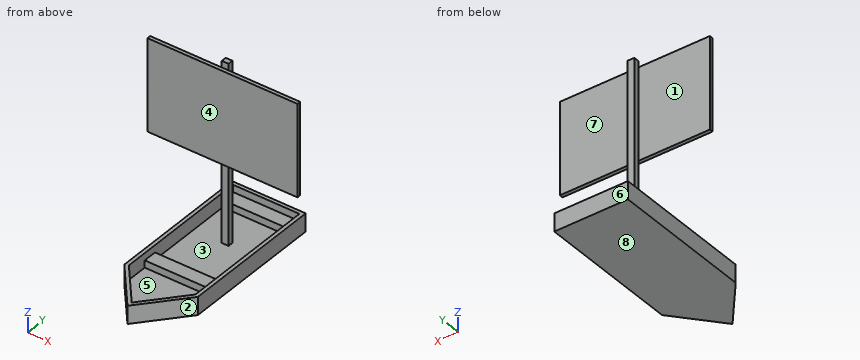
```python
from build123d import *

# Parameters (mm, degrees)
F0_W      = 25.5351066589
F0_H      = 25.5351066589
F0_H_2    = 76.037876308
F0_W_2    = 26.6699995846
F1_DEPTH  = 12.7
F2_T      = -2.54
F3_W      = 47.1251062435
F3_H      = 9.6601096606
F3_H_2    = 9.6465954557
F4_DEPTH  = 5.08
F5_W      = 4.8232972622
F5_H      = 3.6884061992
F6_DEPTH  = 127
F7_W      = 4.8232972622
F7_H      = 2.9607340693
F8_DEPTH  = 2.54
F9_W      = 2.54
F9_H      = 2.9607340693
F10_DEPTH = 50.8
F11_W     = 2.54
F11_H     = 2.9607340693
F12_DEPTH = 50.8
F13_W     = 106.4232972622
F13_H     = 2.54
F14_DEPTH = 62.23


with BuildPart() as f1:
    # F0 (on Top) → F1 (new body)
    with BuildSketch(Plane.XY):
        with Locations((-12.7675533295, -12.7675533295)):
            Rectangle(F0_W, F0_H)
        with Locations((-12.7675533295, 38.018938154)):
            Rectangle(F0_W, F0_H_2)
        with Locations((13.3349997923, 38.018938154)):
            Rectangle(F0_W_2, F0_H_2)
        with Locations((13.3349997923, -12.7675533295)):
            Rectangle(F0_W_2, F0_H)
        Polygon((26.6699995846, -25.5351066589), (0, -25.5351066589), (-25.5351066589, -25.5351066589), (0, -56.4609579742), align=None)
    extrude(amount=F1_DEPTH)

    # F2
    f2_openings = [f1.faces().sort_by_distance(p)[0] for p in [
        (0.542456, 17.179425, 12.7),
    ]]
    offset(amount=F2_T, openings=f2_openings)

    # F3 (on face) → F4 (join)
    with BuildSketch(Plane.XY.offset(2.54)):
        with Locations((0.5674464628, 68.6678214777)):
            Rectangle(F3_W, F3_H)
        with Locations((0.5674464628, -4.8232977279)):
            Rectangle(F3_W, F3_H_2)
    extrude(amount=F4_DEPTH)

    # F5 (on face) → F6 (join)
    with BuildSketch(Plane.XY.offset(2.54)):
        with Locations((-0.1418609172, 37.5933516771)):
            Rectangle(F5_W, F5_H)
    extrude(amount=F6_DEPTH)

    # F7 (on face) → F8 (join)
    with BuildSketch(Plane.XZ.offset(-35.7491485775)):
        with Locations((-0.1418609172, 61.2260736525)):
            Rectangle(F7_W, F7_H)
    extrude(amount=F8_DEPTH)

    # F9 (on face) → F10 (join)
    with BuildSketch(Plane.YZ.offset(2.2697877139)):
        with Locations((34.4791485775, 61.2260736525)):
            Rectangle(F9_W, F9_H)
    extrude(amount=F10_DEPTH)

    # F11 (on face) → F12 (join)
    with BuildSketch(Plane(origin=(-2.5535095483, 0, 0), x_dir=(0, -1, 0), z_dir=(-1, 0, 0))):
        with Locations((-34.4791485775, 61.2260736525)):
            Rectangle(F11_W, F11_H)
    extrude(amount=F12_DEPTH)

    # F13 (on face) → F14 (join)
    with BuildSketch(Plane.XY.offset(62.7064406872)):
        with Locations((-0.1418609172, 34.4791485775)):
            Rectangle(F13_W, F13_H)
    extrude(amount=F14_DEPTH)


solid = f1.part
```
Geometry: final body of the model. Coordinates: model frame, mm. Face numbers are marked on the shaded views. A direction names the side the tool comes from. Round coordinates to 2 decimals unless told otherwise and drop trailing zeros. Order: outer loops, then holes, each group sorted by start corner. A loop starts at its lowest first (then second) coordinate and runs counter-clockwise, first axis right, second up. Notation, with made-up numbers: M 14,82 L 72,82 A17 cw 72,98 Z; hole C 75,72 d8. An arc over 180 degrees is marked long. Use one line per item in the form item = value. Start each with the question number.
Q1. Cut plane B-B (x = 7.5). Return loops of the section in (y, z), and give its area (3 significant figures).
Q2. Mould query, pull axis X, two halves, no side actions, for the marked faces 1, 2 and 3. Classes: +X half, -X half, draft (parallel to the pull), parting line (faces both ways), or undercut.
Q3. Access query for the marked faces 4, 5, 6, 7 and 8. Directions: +Z, -Z, +X, -X, +Y, -Y. A direction counts if a zero-diameter tool reaches every point of the face in a straight line with its end or side. Return the directions, or none.
Q4. Material intervals for line 1 (X direction, y = 57.5, z = 9); line 2 (Y direction, x = 46.5, z = 94); line 3 (Y direction, x = 1.5, z = 118), sorted ascending. Write a range as [from, to].
Q5. Cut plane C-C (y = -16.5). Return loops of the section in (x, z).
Q6. Pin query (flat end, axial travel): pin 1 Ø6 at (x, y) = (5.5, -36.5) entering from +Z; pin 2 Ø6 at (y, z) = (37, 46.5) entering from +X; pin 3 Ø5 at (x, y) = (14, -5.5) entering from -Z; pin 4 Ø11 at (y, z) = (20, 5) entering from -X. Return the tip coordinate at first contact, or that it passes through.
Q7. Cut plane A-A (z = 98.5). Return loops of the section in (x, y).
Q8. Cut plane D-D (x = -43). Return loops of the section in (y, z), and give its area (3 significant figures).
Geometry results:
q1.outline = M -47.76,0 L 76.04,0 L 76.04,12.7 L 73.5,12.7 L 73.5,7.62 L 63.84,7.62 L 63.84,2.54 L 0,2.54 L 0,7.62 L -9.65,7.62 L -9.65,2.54 L -43.87,2.54 L -43.87,12.7 L -47.76,12.7 Z; M 33.21,59.75 L 35.75,59.75 L 35.75,124.94 L 33.21,124.94 Z
q1.area = 643 mm^2
q2.face_1 = draft
q2.face_2 = +X half
q2.face_3 = undercut
q3.face_4 = +Z, +X, -X, -Y
q3.face_5 = +Z
q3.face_6 = +Z, -Z, +X, -X, +Y
q3.face_7 = +Z, +X, +Y
q3.face_8 = -Z, +X, -X, +Y, -Y
q4.line_1 = [-25.54, -23], [24.13, 26.67]
q4.line_2 = [33.21, 35.75]
q4.line_3 = [33.21, 39.44]
q5.outline = M -25.54,0 L 26.67,0 L 26.67,12.7 L 24.13,12.7 L 24.13,2.54 L -23,2.54 L -23,12.7 L -25.54,12.7 Z
q6.pin_1 = 2.54
q6.pin_2 = 2.27
q6.pin_3 = 0
q6.pin_4 = -25.54
q7.outline = M -53.35,33.21 L 53.07,33.21 L 53.07,35.75 L 2.27,35.75 L 2.27,39.44 L -2.55,39.44 L -2.55,35.75 L -53.35,35.75 Z
q8.outline = M 33.21,59.75 L 35.75,59.75 L 35.75,124.94 L 33.21,124.94 Z
q8.area = 166 mm^2
